from build123d import *

# Parameters (mm, degrees)
SKETCH1_R           = 2.25
BOSS_EXTRUDE1_DEPTH = 5


with BuildPart() as part:
    # Sketch1 → Boss-Extrude1 (new body)
    with BuildSketch(Plane(origin=(0, 0, 0), x_dir=(1, 0, 0), z_dir=(0, 1, 0))):
        with BuildLine():
            Line((-5.893587617, -1.125), (-4.420190713, -8.84375))
            ThreePointArc((-4.420190713, -8.84375), (0, -12.5), (4.420190713, -8.84375))
            Line((4.420190713, -8.84375), (5.893587617, -1.125))
            ThreePointArc((5.893587617, -1.125), (0, 6), (-5.893587617, -1.125))
        make_face()
        with Locations(Location((0, -8, 0), (0, 0, 270))):
            Circle(SKETCH1_R, mode=Mode.SUBTRACT)
        Polygon((0, 4.041451884), (-3.5, 2.020725942), (-3.5, -2.020725942), (0, -4.041451884), (3.5, -2.020725942), (3.5, 2.020725942), align=None, mode=Mode.SUBTRACT)
    extrude(amount=BOSS_EXTRUDE1_DEPTH)


solid = part.part
Read the model definition and answer for the solid it produces. Units are mm, in the model's axes. A direction names the side the tool comes from. Coordinates: 2 decimals unless noted, no trailing zeros. Loops run counter-clockwise (first coordinate to the right, second up) from the corner with the lowest first, then second, coordinate; pieces in that order, holes last. Notation, with made-up numbers: (14, 71) - (19, 71) arc R22 ccw to (19, 85) - close; hole circle Ø10 at (88, -16.75). An arc over 180 degrees is marked (long way). Answer in a Markdown table with one row per item.
Q1. For faces 1 (the flat face through (0, 5, 5)), 2 (the flat face through (3.5, 2, 0)), determine the directions among +Z, -Z, +X, -X, +Y, -Y from which every point of the face is accessible in a straight line to the end or side of a thin tool.
Here are the results:
| item | result |
|---|---|
| face 1 | +Z, -Z, +X, -X, +Y |
| face 2 | +Y, -Y |
Q2. Find section A-A on y = 1.45. Write down the section's boundary in (x, z) (3 decimals).
Here are the results:
| item | result |
|---|---|
| outline | (-5.894, 1.125) arc R6 ccw (long way) to (5.894, 1.125) - (4.42, 8.844) arc R4.5 ccw to (-4.42, 8.844) - close; hole (-3.5, -2.021) - (0, -4.041) - (3.5, -2.021) - (3.5, 2.021) - (0, 4.041) - (-3.5, 2.021) - close; hole circle Ø4.5 at (0, 8) |
Q3. Given P1, Ø1, axis at y = 3.5, z = 4.5, coming from the +X side; P2, Ø1, axis at x = 2.5, y = 2.5, coming from the +Z side; P3, Ø7, axis at x = 0, z = 8, coming from the -Y side; P4, Ø2, axis at y = 3, z = 3.5, coming from the -X side, each flat-ended and moving along its own axis, determine where each tip first touches the part or whether it passes through.
Here are the results:
| item | result |
|---|---|
| P1 | stops at x = 5.34 |
| P2 | stops at z = 12.03 |
| P3 | stops at y = 0 |
| P4 | stops at x = -5.63 |
Q4. Find section D-D on z = -3.25. Write down the section's boundary in (x, y), plus the area to 3 significant figures.
Here are the results:
| item | result |
|---|---|
| outline | (-5.04, 0) - (-1.37, 0) - (-1.37, 5) - (-5.04, 5) - close; (1.37, 0) - (5.04, 0) - (5.04, 5) - (1.37, 5) - close |
| area | 36.7 mm^2 |
Q5. Find section C-C on x = 0.25. Write down the section's boundary in (y, z), plus the area to 3 significant figures.
Here are the results:
| item | result |
|---|---|
| outline | (0, -5.99) - (5, -5.99) - (5, -3.9) - (0, -3.9) - close; (0, 3.9) - (5, 3.9) - (5, 5.76) - (0, 5.76) - close; (0, 10.24) - (5, 10.24) - (5, 12.49) - (0, 12.49) - close |
| area | 31.1 mm^2 |
Q6. Straight lines are drawn through the part: line 1 along Z through (x, y) = (1, 2.2); line 2 along X through (y, z) = (1.95, -2.25); line 3 along X through (y, z) = (1.55, 8). For each, find the intervals that lie inside material, in ascending order. Write a range as [from, to].
Here are the results:
| item | result |
|---|---|
| line 1 | z = [-5.92, -3.46], [3.46, 5.98], [10.02, 12.39] |
| line 2 | x = [-5.56, -3.1], [3.1, 5.56] |
| line 3 | x = [-4.58, -2.25], [2.25, 4.58] |
Q7. The mould has two halves that part along X. Classify faces 3 (the flat face through (-5.167, 2.465, 4.93)), 4 (the flat face through (0, 0, 5)), 5 (the flat face through (1.726, 2.465, 3.045)), 6 (the cylindrical face through (-0.1, 2.5, 12.5)): pulls with the +X half, pulls with the -X half, needs draft (parallel to the pull), parting line crosses it, or undercut.
Here are the results:
| item | result |
|---|---|
| face 3 | pulls with the -X half |
| face 4 | needs draft |
| face 5 | undercut |
| face 6 | parting line crosses it |
Q8. Find section B-B on z = 0. Write down the section's boundary in (x, y), plus the area to 3 significant figures.
Here are the results:
| item | result |
|---|---|
| outline | (-6, 0) - (-3.5, 0) - (-3.5, 5) - (-6, 5) - close; (3.5, 0) - (6, 0) - (6, 5) - (3.5, 5) - close |
| area | 25.0 mm^2 |
